from build123d import *

# Parameters (mm, degrees)
F1_DEPTH = 76.2
F2_T     = -6.35
F3_R     = 6.35
F4_DEPTH = 609.6
F6_D     = 12.7


with BuildPart() as f1:
    # F0 (on Top) → F1 (new body)
    with BuildSketch(Plane.XY):
        Polygon((-304.8, 304.8), (-304.8, -304.8), (304.8, -304.8), (304.8, -228.6), (-228.6, -228.6), (-228.6, 228.6), (304.8, 228.6), (304.8, 304.8), align=None)
    extrude(amount=F1_DEPTH)

    # F2
    f2_openings = [f1.faces().sort_by_distance(p)[0] for p in [
        (304.8, -266.7, 38.1),
        (304.8, 266.7, 38.1),
    ]]
    offset(amount=F2_T, openings=f2_openings, kind=Kind.INTERSECTION)

    # F3 (on face) → F4 (join)
    with BuildSketch(Plane.XZ.offset(304.8)):
        with Locations((-179.052978754, 31.5465517342)):
            Circle(F3_R)
    extrude(amount=-F4_DEPTH)

    # F6 (through all)
    with Locations(Plane(origin=(0, 304.8, 0), x_dir=(-1, 0, 0), z_dir=(0, 1, 0))):
        with Locations((-254, 38.1), (-101.6, 38.1)):
            Hole(F6_D / 2)


solid = f1.part
Verification items for the finished model (mm, model axes). A direction names the side the tool comes from. Coordinates: 2 decimals unless noted, no trailing zeros. Order: outer loops, then holes, each group sorted by start corner. A loop starts at its lowest first (then second) coordinate and runs counter-clockwise, first axis right, second up. Notation, with made-up numbers: M 38,33.25 L 62,33.25 A10 cw 62,51.25 Z; hole C 22,-20.75 d5. An arc over 180 degrees is marked long. One line per item, written item: value. Start each with the question number.
Item 1: Sectioned sample at A-A (z = 15). Enter the section's corners in (x, y), then the cut area to 3 significant figures.
Item 2: Scan lines: probe 1 along Y at (x, z) = (44, 10); probe 2 along X at (y, z) = (-111.5, 24.5). Record each from-to range of solid material in increasing order.
Item 3: Sectioned sample at B-B (x = -78.5). Enter the section's corners in (y, z).
Item 4: Sectioned sample at D-D (y = 244). Enter the section's corners in (x, z), then the cut area to 3 significant figures.
Item 5: Access from +Z, -Z, +X, -X, +Y, -Y to the whole of each face (thin tool, end or side, straight path). Record for faces 1 (the flat face through (-298.45, 4, 38)), 2 (the flat face through (-228.6, -3, 38)), 3 (the flat face through (304.8, -267, 71)).
Item 6: Mould release check, pull along X, two halves, no side actions. Record for faces 4 (the flat face through (-250, 1, 0)), 5 (the flat face through (-244, 1, 69.85)), 6 (the flat face through (-304.8, 4, 38)): released by +X, released by -X, zero draft, split by the parting line, or undercut.
Item 7: Gauge pin test, flat ends, axial feed: pin 1 (16.5 mm diameter, centred on x = 101.6, z = 38.1, fed in from +Y); pin 2 (3 mm diameter, centred on y = 189, z = 50.5, fed in from +X). Record the tip position at first contact, or that the pin passes through.
Item 8: Sectioned sample at C-C (y = -47). Enter the section's corners in (x, z).
Conclusion:
1. outline: M -304.8,-304.8 L 304.8,-304.8 L 304.8,-298.45 L -298.45,-298.45 L -298.45,298.45 L 304.8,298.45 L 304.8,304.8 L -304.8,304.8 Z; M -234.95,-234.95 L 304.8,-234.95 L 304.8,-228.6 L -228.6,-228.6 L -228.6,228.6 L 304.8,228.6 L 304.8,234.95 L -234.95,234.95 Z
1. area: 21,300 mm^2
2. probe 1: y = -304.8 to -298.45, -234.95 to -228.6, 228.6 to 234.95, 298.45 to 304.8
2. probe 2: x = -304.8 to -298.45, -234.95 to -228.6
3. outline: M -304.8,0 L -228.6,0 L -228.6,76.2 L -304.8,76.2 Z; M 228.6,0 L 304.8,0 L 304.8,76.2 L 228.6,76.2 Z; hole M -298.45,6.35 L -234.95,6.35 L -234.95,69.85 L -298.45,69.85 Z; hole M 234.95,6.35 L 298.45,6.35 L 298.45,69.85 L 234.95,69.85 Z
4. outline: M -304.8,0 L 304.8,0 L 304.8,6.35 L -298.45,6.35 L -298.45,69.85 L 304.8,69.85 L 304.8,76.2 L -304.8,76.2 Z; C -179.05,31.55 d12.7
4. area: 8,270 mm^2
5. face 1: none
5. face 2: +Z, -Z
5. face 3: +Z, -Z, +X, +Y, -Y
6. face 4: zero draft
6. face 5: undercut
6. face 6: released by -X
7. pin 1: stops at y = 304.8
7. pin 2: stops at x = -228.6
8. outline: M -304.8,0 L -228.6,0 L -228.6,76.2 L -304.8,76.2 Z; C -179.05,31.55 d12.7; hole M -298.45,6.35 L -234.95,6.35 L -234.95,69.85 L -298.45,69.85 Z
